Model file for the job. Use its own axes, mm. Round coordinates to 2 decimals unless told otherwise and drop trailing zeros. Order: outer loops, then holes, each group sorted by start corner. A loop starts at its lowest first (then second) coordinate and runs counter-clockwise, first axis right, second up. Notation, with made-up numbers: (32, 70) - (56, 70) arc R8 ccw to (56, 83) - close; hole circle Ø5 at (50.25, -18.75). An arc over 180 degrees is marked (long way). Write item = value, one per line.
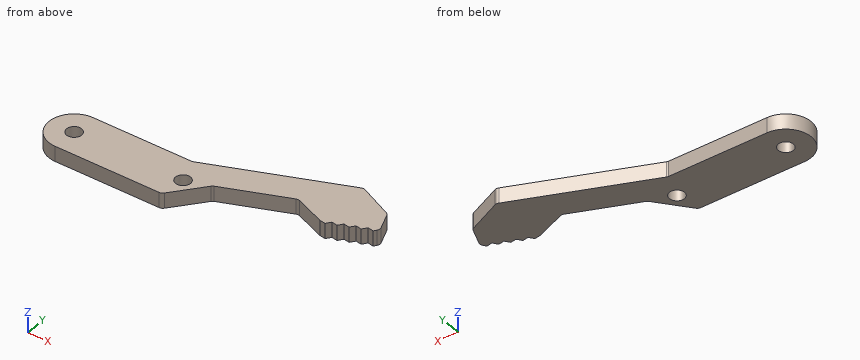
```python
from build123d import *

# Parameters (mm, degrees)
SKETCH1_R           = 1.5
BOSS_EXTRUDE1_DEPTH = 3
FILLET1_R           = 1


with BuildPart() as part:
    # Sketch1 → Boss-Extrude1 (new body)
    with BuildSketch(Plane.XY):
        with BuildLine():
            Line((20.05, 5), (0, 5))
            ThreePointArc((0, 5), (-5, 0), (0, -5))
            Line((0, -5), (21.474824475, -5))
            Line((21.474824475, -5), (26.72989842, 1.621129525))
            Line((26.72989842, 1.621129525), (39.900164389, 7.036080522))
            Line((39.900164389, 7.036080522), (46.188488025, 4.540007042))
            Line((46.188488025, 4.540007042), (47.351030887, 4.342221563))
            Line((47.351030887, 4.342221563), (48.038244482, 5.300533868))
            Line((48.038244482, 5.300533868), (49.200787343, 5.102748388))
            Line((49.200787343, 5.102748388), (49.888000938, 6.061060693))
            Line((49.888000938, 6.061060693), (51.050543799, 5.863275214))
            Line((51.050543799, 5.863275214), (51.737757394, 6.821587519))
            Line((51.737757394, 6.821587519), (52.900300256, 6.623802039))
            Line((52.900300256, 6.623802039), (53.587513851, 7.582114344))
            Line((53.587513851, 7.582114344), (54.750056712, 7.384328864))
            Line((54.750056712, 7.384328864), (55.437270307, 8.34264117))
            Line((55.437270307, 8.34264117), (53.72608495, 12.504593197))
            Line((53.72608495, 12.504593197), (46.409029503, 15.837507263))
            Line((46.409029503, 15.837507263), (20.05, 5))
        make_face()
        Circle(SKETCH1_R, mode=Mode.SUBTRACT)
        with Locations((22, 0)):
            Circle(SKETCH1_R, mode=Mode.SUBTRACT)
    extrude(amount=BOSS_EXTRUDE1_DEPTH)

    # Fillet1
    fillet1_edges = [part.edges().sort_by_distance(p)[0] for p in [
        (21.474824475, -5, 1.5),
        (20.05, 5, 1.5),
        (46.409029503, 15.837507263, 1.5),
        (53.72608495, 12.504593197, 1.5),
        (55.437270307, 8.34264117, 1.5),
        (46.188488025, 4.540007042, 1.5),
        (39.900164389, 7.036080522, 1.5),
        (26.72989842, 1.621129525, 1.5),
    ]]
    fillet(fillet1_edges, radius=FILLET1_R)


solid = part.part
```
1) Wall check: line 1 along Y through (x, z) = (0, 1.05); line 2 along Y through (x, z) = (2.5, 0.8); line 3 along Y through (x, z) = (22, 1.2). Give the ranges that are in metal, low to high.
Conclusion:
line_1 = -5 to -1.5, 1.5 to 5
line_2 = -5 to 5
line_3 = -4.34 to -1.5, 1.5 to 5.8
2) Cut at A-A (y = 0.75). Write the cut outline in (x, z), and give its area (3 significant figures).
Conclusion:
outline = (-4.94, 0) - (-1.3, 0) - (-1.3, 3) - (-4.94, 3) - close; (1.3, 0) - (20.7, 0) - (20.7, 3) - (1.3, 3) - close; (23.3, 0) - (26.04, 0) - (26.04, 3) - (23.3, 3) - close
area = 77.4 mm^2
3) Cut at B-B (z = 0.75). Give the number of separate pieces and of enclosed holes in the cut face, and give its area (3 significant figures).
Conclusion:
separate_pieces = 1
enclosed_holes = 2
area = 488 mm^2
4) Flat gauge pin, fed straight in: pin 1 Ø3.5 at (x, y) = (22, 0) entering from +Z. Where does the tip first touch, or does it go through?
Conclusion:
pin_1 = 3
5) Cut at D-D (x = 42.5). Write the cut outline in (y, z).
Conclusion:
outline = (6, 0) - (14.23, 0) - (14.23, 3) - (6, 3) - close
6) Cut at C-C (x = 18.5). Write the cut outline in (y, z), and give its area (3 significant figures).
Conclusion:
outline = (-5, 0) - (5, 0) - (5, 3) - (-5, 3) - close
area = 30.0 mm^2
